Verification items for the finished model (mm, model axes). A direction names the side the tool comes from. Coordinates: 2 decimals unless noted, no trailing zeros. Write each loop counter-clockwise with the first axis right and the second up, starting at its lowest first coordinate (ties: lowest second). Pieces come first, ordered by that corner, then holes. Notation, with made-up numbers: (65, 29) - (88, 29) arc R23 cw to (88, 42) - close; hole circle Ø2 at (-9.5, 65.5). An arc over 180 degrees is marked (long way). Use one line per item in the form item = value. Start each with the question number.
(1) Sectioned sample at B-B (y = -11). Record the cut outline in (x, z), and give its area (3 significant figures).
(2) Tool access check on faces 1 (the cylindrical face through (-8.95, 0.13, 7.47)), 2 (the flat face through (-7, -13.335, 0)), 3 (the flat face through (-3.219, -0.187, 5.474)). Record the directions out of +Z, -Z, +X, -X, +Y, -Y that give a thin tool (end or side, any length) a straight path to the whole face; none if there is none.
(3) Mould release check, pull along X, two halves, no side actions. Record for faces 4 (the flat face through (-3.131, -0.187, -5.525)), 5 (the cylindrical face through (-11.657, 0.133, -0.03)), 6 (the cylindrical face through (5.855, 0.133, -10.08)), 7 (the cylindrical face through (11.657, 0.133, 0.03)): released by +X, released by -X, zero draft, split by the parting line, or undercut.
(4) Sectioned sample at C-C (z = 4.5). Record the cut outline in (x, y) (3 decimals).
(5) Sectioned sample at A-A (z = 0). Record the cut outline in (x, y) (3 decimals), and give its area (3 significant figures).
(6) Material ranges on line 1 (Y direction, x = -12, z = 0) (3 decimals); line 2 (X direction, y = -7.5, z = 10.5); line 3 (X direction, y = -8, z = -0.5), recorded low to high. Write a range as [from, to].
(7) Gauge pin test, flat ends, axial feed: pin 1 Ø2 at (x, y) = (7, 9) entering from -Z; pin 2 Ø12 at (x, y) = (-7.5, 2) entering from +Z; pin 3 Ø12 at (y, z) = (-10.5, 8.5) entering from +X. Record the tip position at first contact, or that the pin passes through.
from build123d import *

# Parameters (mm, degrees)
MOUNTINGHOLES_R         = 14.323949
BOSS_EXTRUDE1_DEPTH     = 9.525
CUT_EXTRUDE1_DEPTH      = 19.05
CIRPATTERN1_COUNT       = 18
FLANGE_R                = 16.228949
BOSS_EXTRUDE2_DEPTH     = 3.81
BOSS_EXTRUDE3_START     = 3.81
SKETCH6_R               = 16.228949
BOSS_EXTRUDE3_DEPTH     = 3.81
CUT_EXTRUDE5_DEPTH      = 32.512
CUT_EXTRUDE5_DEPTH_BACK = 31.242


with BuildPart() as part:
    # mountingHoles → Boss-Extrude1 (new, symmetric)
    with BuildSketch(Plane(origin=(0, 0, 0), x_dir=(1, 0, 0), z_dir=(0, 1, 0))):
        with Locations(Location((0, 0, 0), (0, 0, 90))):
            Circle(MOUNTINGHOLES_R)
    extrude(amount=BOSS_EXTRUDE1_DEPTH, both=True)

    # Sketch2 → Cut-Extrude1 (cut)
    with BuildSketch(Plane(origin=(0, 9.525, 0), x_dir=(1, 0, 0), z_dir=(0, 1, 0))):
        with BuildLine():
            Line((0, 13.460349), (0, 14.323949))
            ThreePointArc((0, 14.323949), (2.487327641, 14.106336029), (4.89907909, 13.460109176))
            Line((4.89907909, 13.460109176), (4.603710494, 12.648590629))
            ThreePointArc((4.603710494, 12.648590629), (4.430828603, 12.710183047), (4.257123016, 12.769412627))
            ThreePointArc((4.257123016, 12.769412627), (3.925929741, 12.745227134), (3.709846002, 12.493072933))
            ThreePointArc((3.709846002, 12.493072933), (2.024207951, 11.479853752), (0.786767683, 13.008490507))
            ThreePointArc((0.786767683, 13.008490507), (0.669957204, 13.319342941), (0.367009253, 13.455344641))
            ThreePointArc((0.367009253, 13.455344641), (0.183521685, 13.459097852), (0, 13.460349))
        make_face()
    cut_extrude1 = extrude(amount=-CUT_EXTRUDE1_DEPTH, mode=Mode.SUBTRACT)

    # CirPattern1: Cut-Extrude1 ×18 about axis
    cirpattern1_axis = Axis((0, 0, 0), (0, 1, 0))
    for i in range(1, CIRPATTERN1_COUNT):
        add(cut_extrude1.rotate(cirpattern1_axis, i * 360 / CIRPATTERN1_COUNT), mode=Mode.SUBTRACT)

    # flange → Boss-Extrude2 (add)
    with BuildSketch(Plane(origin=(0, 9.525, 0), x_dir=(1, 0, 0), z_dir=(0, 1, 0))):
        with Locations(Location((0, 0, 0), (0, 0, 90))):
            Circle(FLANGE_R)
    extrude(amount=BOSS_EXTRUDE2_DEPTH)

    # Sketch6 → Boss-Extrude3 (add)
    with BuildSketch(Plane.XZ.offset(9.525).offset(BOSS_EXTRUDE3_START)):
        with Locations(Location((0, 0, 0), (0, 0, 270))):
            Circle(SKETCH6_R)
    extrude(amount=-BOSS_EXTRUDE3_DEPTH)

    # Sketch1_5 → Cut-Extrude5 (cut, two sides: drawn at the far end of the back side and taken through both)
    with BuildSketch(Plane(origin=(0, 0, 0), x_dir=(1, 0, 0), z_dir=(0, 1, 0)).offset(-CUT_EXTRUDE5_DEPTH_BACK)):
        Polygon((0, 7.332348419), (-6.35, 3.666174209), (-6.35, -3.666174209), (0, -7.332348419), (6.35, -3.666174209), (6.35, 3.666174209), align=None)
    extrude(amount=CUT_EXTRUDE5_DEPTH + CUT_EXTRUDE5_DEPTH_BACK, mode=Mode.SUBTRACT)


solid = part.part
Answers below:
q1.outline = circle Ø32.46 at (0, 0); hole (-6.35, -3.67) - (0, -7.33) - (6.35, -3.67) - (6.35, 3.67) - (0, 7.33) - (-6.35, 3.67) - close
q1.area = 688 mm2
q2.face_1 = none
q2.face_2 = +Z, -Z, +X, -X, -Y
q2.face_3 = +Y, -Y
q3.face_4 = undercut
q3.face_5 = released by -X
q3.face_6 = undercut
q3.face_7 = released by +X
q4.outline = (-15.593, -13.335) - (-4.906, -13.335) - (-4.906, 13.335) - (-15.593, 13.335) - (-15.593, 9.525) - (-10.864, 9.525) - (-10.864, -9.525) - (-15.593, -9.525) - close; (4.906, -13.335) - (15.593, -13.335) - (15.593, -9.525) - (10.864, -9.525) - (10.864, 9.525) - (15.593, 9.525) - (15.593, 13.335) - (4.906, 13.335) - close
q5.outline = (-16.229, -13.335) - (-6.35, -13.335) - (-6.35, 13.335) - (-16.229, 13.335) - (-16.229, 9.525) - (-11.657, 9.525) - (-11.657, -9.525) - (-16.229, -9.525) - close; (6.35, -13.335) - (16.229, -13.335) - (16.229, -9.525) - (11.657, -9.525) - (11.657, 9.525) - (16.229, 9.525) - (16.229, 13.335) - (6.35, 13.335) - close
q5.area = 353 mm2
q6.line_1 = [-13.335, -9.525], [9.525, 13.335]
q6.line_2 = [-8.42, -7.78], [-5.37, 5.37], [7.78, 8.42]
q6.line_3 = [-11.74, -6.35], [6.35, 11.74]
q7.pin_1 = -15.02
q7.pin_2 = 12.79
q7.pin_3 = 16.04
